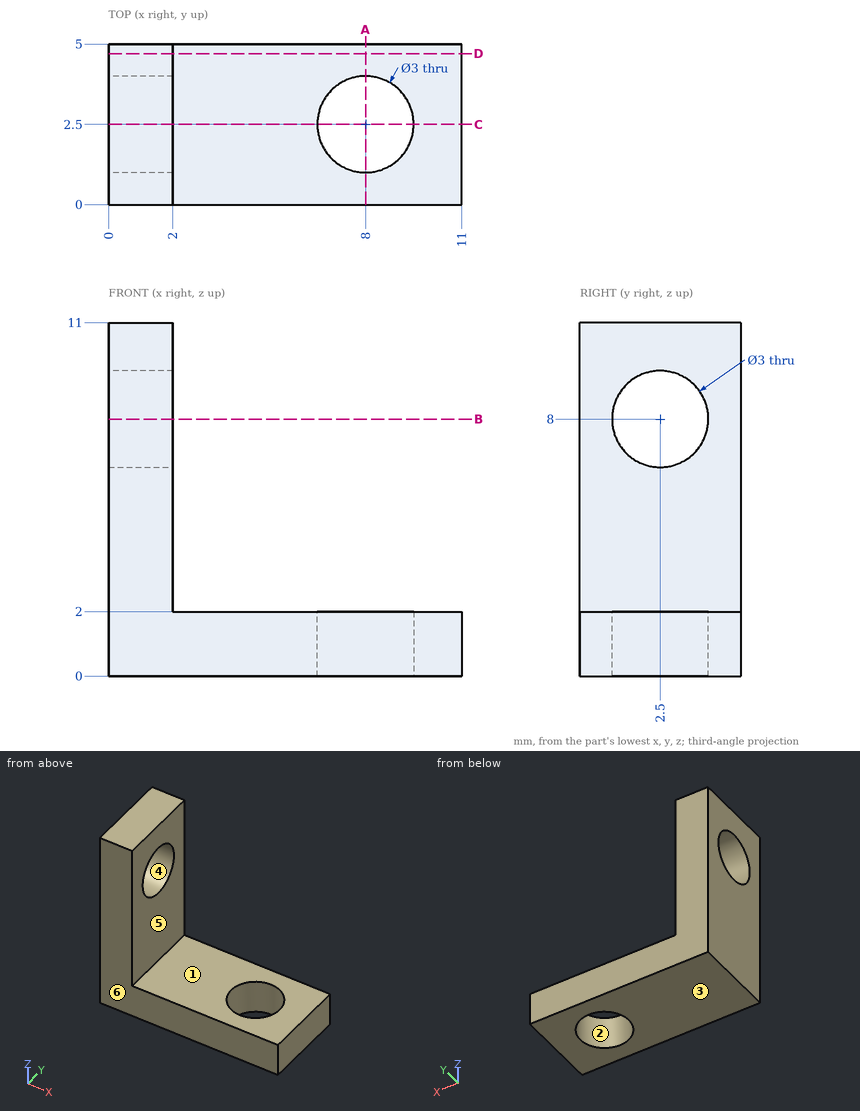
Input: dimensioned drawing with shaded views. Units: mm. Origin: part minimum x, y, z. A direction names the side the tool comes from. Give positions to 0.01 mm unless a question says otherwise; leave off trailing zeros. Write each loop counter-clockwise with the first axis right and the second up, starting at its lowest first coordinate (ties: lowest second). Pieces come first, ordered by that corner, then holes.
1. Pull-direction query (Z, two-part tool) for the marked faces 1, 2, 3 and 4; classes: +Z half, -Z half, draft (parallel to the pull), parting line (faces both ways), or undercut.
2. Section query A-A (x = 8). Return the cut outline in (y, z).
3. Material intervals for line 1 along Y through (x, z) = (1.5, 8); line 2 along X through (y, z) = (3.55, 4), sorted ascending.
4. Access query for the marked faces 5 and 6. Directions: +Z, -Z, +X, -X, +Y, -Y. A direction counts if a zero-diameter tool reaches every point of the face in a straight line with its end or side. Return the directions, or none.
5. Section query B-B (z = 8). Return the cut outline in (x, y).
6. Section query D-D (y = 4.7). Return the cut outline in (x, z), then the cut area to 3 significant figures.
7. Section query C-C (y = 2.5). Return the cut outline in (x, z), then the cut area to 3 significant figures.
8. First-contact query: pin 1 (1.5 mm diameter, centred on y = 1.5, z = 3.5, fed in from +X); pin 2 (2.5 mm diameter, centred on x = 6.5, y = 1.5, fed in from +Z); pin 3 (2.5 mm diameter, centred on x = 8, y = 2.5, fed in from +Z). Flat tips, straight axial feed; report the tip coordinate or a pass-through.
Output values:
1. face 1: +Z half
1. face 2: draft
1. face 3: -Z half
1. face 4: undercut
2. outline: (0, 0) - (1, 0) - (1, 2) - (0, 2) - close; (4, 0) - (5, 0) - (5, 2) - (4, 2) - close
3. line 1: y = 0 to 1, 4 to 5
3. line 2: x = 0 to 2
4. face 5: +Z, +X, +Y, -Y
4. face 6: +Z, -Z, +X, -X, -Y
5. outline: (0, 0) - (2, 0) - (2, 1) - (0, 1) - close; (0, 4) - (2, 4) - (2, 5) - (0, 5) - close
6. outline: (0, 0) - (11, 0) - (11, 2) - (2, 2) - (2, 11) - (0, 11) - close
6. area: 40.0 mm2
7. outline: (0, 0) - (6.5, 0) - (6.5, 2) - (2, 2) - (2, 6.5) - (0, 6.5) - close; (0, 9.5) - (2, 9.5) - (2, 11) - (0, 11) - close; (9.5, 0) - (11, 0) - (11, 2) - (9.5, 2) - close
7. area: 28.0 mm2
8. pin 1: stops at x = 2
8. pin 2: stops at z = 2
8. pin 3: passes through
